Geometry: see drawing. Coordinates: mm, zero at the bounding-box minimum. Coordinates: 2 decimals unless noted, no trailing zeros. Loops run counter-clockwise (first coordinate to the right, second up) from the corner with the lowest first, then second, coordinate; pieces in that order, holes last. Notation, with made-up numbers: (75, -18) -> (115, -18) arc R6 cw to (115, -9) -> close; hole circle Ø1 at (59, 12). An arc over 180 degrees is marked (long way). Put each result on its own line as item: value. Start each with the question number.
1) Cut plane C-C (x = 16). Return the cut outline in (y, z).
2) Cut plane D-D (z = 46). Return the cut outline in (x, y), plus the area to 3 significant figures.
3) Material intervals for L1, parallel to Y at x = 48, z = 22; L2, parallel to X at y = 8.5, z = 23; L3, parallel to X at y = 7.5, z = 39, sorted ascending.
4) Cut plane B-B (z = 10). Return the cut outline in (x, y).
5) Cut plane A-A (y = 8). Return the cut outline in (x, z).
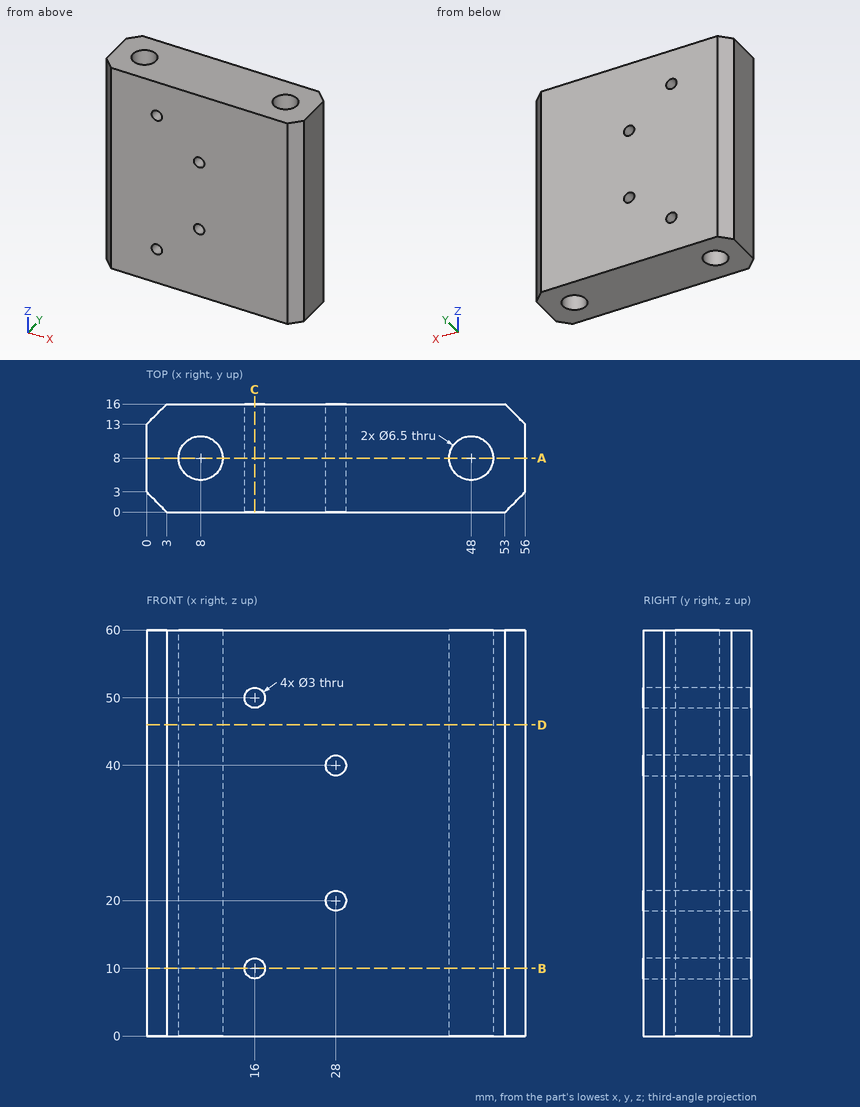
Results found:
1. outline: (0, 0) -> (16, 0) -> (16, 8.5) -> (0, 8.5) -> close; (0, 11.5) -> (16, 11.5) -> (16, 48.5) -> (0, 48.5) -> close; (0, 51.5) -> (16, 51.5) -> (16, 60) -> (0, 60) -> close
2. outline: (0, 3) -> (3, 0) -> (53, 0) -> (56, 3) -> (56, 13) -> (53, 16) -> (3, 16) -> (0, 13) -> close; hole circle Ø6.5 at (8, 8); hole circle Ø6.5 at (48, 8)
2. area: 812 mm2
3. L1: y = 0 to 4.75, 11.25 to 16
3. L2: x = 0 to 4.79, 11.21 to 44.79, 51.21 to 56
3. L3: x = 0 to 4.79, 11.21 to 26.88, 29.12 to 44.79, 51.21 to 56
4. outline: (0, 3) -> (3, 0) -> (14.5, 0) -> (14.5, 16) -> (3, 16) -> (0, 13) -> close; (17.5, 0) -> (53, 0) -> (56, 3) -> (56, 13) -> (53, 16) -> (17.5, 16) -> close; hole circle Ø6.5 at (8, 8); hole circle Ø6.5 at (48, 8)
5. outline: (0, 0) -> (4.75, 0) -> (4.75, 60) -> (0, 60) -> close; (11.25, 0) -> (44.75, 0) -> (44.75, 60) -> (11.25, 60) -> close; (51.25, 0) -> (56, 0) -> (56, 60) -> (51.25, 60) -> close; hole circle Ø3 at (16, 10); hole circle Ø3 at (16, 50); hole circle Ø3 at (28, 20); hole circle Ø3 at (28, 40)
